Design review of the part built by this model. Coordinates are the model's own, in mm. A direction names the side the tool comes from. Give positions to 0.01 mm unless a question says otherwise; leave off trailing zeros. Order: outer loops, then holes, each group sorted by start corner. A loop starts at its lowest first (then second) coordinate and runs counter-clockwise, first axis right, second up. Notation, with made-up numbers: M 16.25,60.25 L 50.25,60.25 A18 ccw 50.25,69.25 Z; hole C 14.5,85.5 d8. An arc over 180 degrees is marked long. Answer as a JSON object with one key per item and string values.
from build123d import *

# Parameters (mm, degrees)
SKETCH1_R           = 30
SKETCH1_R_2         = 7
BOSS_EXTRUDE1_DEPTH = 10
CUT_EXTRUDE1_DEPTH  = 21
FILLET1_R           = 30
FILLET2_R           = 55


with BuildPart() as part:
    # Sketch1 → Boss-Extrude1 (new body, symmetric)
    with BuildSketch(Plane(origin=(0, 0, 0), x_dir=(1, 0, 0), z_dir=(0, 1, 0))):
        with BuildLine():
            Line((128.063755469, 9.084385863), (27.935473676, 25.760615491))
            ThreePointArc((27.935473676, 25.760615491), (-38, 0), (27.935473676, -25.760615491))
            Line((27.935473676, -25.760615491), (128.063755469, -9.084385863))
            ThreePointArc((128.063755469, -9.084385863), (155, 0), (128.063755469, 9.084385863))
        make_face()
        Circle(SKETCH1_R, mode=Mode.SUBTRACT)
        with Locations((140, 0)):
            Circle(SKETCH1_R_2, mode=Mode.SUBTRACT)
    extrude(amount=BOSS_EXTRUDE1_DEPTH, both=True)

    # Sketch2 → Cut-Extrude1 (cut, through all)
    with BuildSketch(Plane(origin=(0, 10, 0), x_dir=(1, 0, 0), z_dir=(0, 1, 0))):
        with BuildLine():
            Line((44.461373165, 15.911828816), (101.502639752, 6.411683174))
            ThreePointArc((101.502639752, 6.411683174), (106.934782609, 0), (101.502639752, -6.411683174))
            Line((101.502639752, -6.411683174), (44.461373165, -15.911828816))
            ThreePointArc((44.461373165, -15.911828816), (39.963398771, -14.368423983), (38.791061861, -9.759790965))
            ThreePointArc((38.791061861, -9.759790965), (40, 0), (38.791061861, 9.759790965))
            ThreePointArc((38.791061861, 9.759790965), (39.963398771, 14.368423983), (44.461373165, 15.911828816))
        make_face()
    extrude(amount=-CUT_EXTRUDE1_DEPTH, mode=Mode.SUBTRACT)

    # Fillet1
    fillet1_edges = [part.edges().sort_by_distance(p)[0] for p in [
        (128.063755469, 0, 9.084385863),
        (128.063755469, 0, -9.084385863),
    ]]
    fillet(fillet1_edges, radius=FILLET1_R)

    # Fillet2
    fillet2_edges = [part.edges().sort_by_distance(p)[0] for p in [
        (27.935473676, 0, 25.760615491),
        (27.935473676, 0, -25.760615491),
    ]]
    fillet(fillet2_edges, radius=FILLET2_R)


solid = part.part
(1) Insertion check: pin 1 (4 mm diameter, centred on x = 29, y = 5, fed in from -Z); pin 2 (5 mm diameter, centred on x = 71, y = 6.5, fed in from -Z); pin 3 (1 mm diameter, centred on y = 2, z = 21, fed in from -X). Each pin has a flat end and moves straight along its axis. Give the tip position at first contact, or say it passes through.
Checked values:
{"pin 1": "stops at z = -28.25", "pin 2": "stops at z = -19", "pin 3": "stops at x = -32"}
(2) We need section C-C (y = -8). Write out the cut boundary in (x, z).
Checked values:
{"outline": "M 20.92,-31.73 A55 cw 42.15,-23.39 L 115.89,-11.11 A30 cw 133.6,-13.57 A15 ccw long 133.6,13.57 A30 cw 115.89,11.11 L 42.15,23.39 A55 cw 20.92,31.73 A38 ccw long Z; hole C 0,0 d60; hole M 38.79,-9.76 A5 ccw 44.46,-15.91 L 101.5,-6.41 A6.5 ccw 101.5,6.41 L 44.46,15.91 A5 ccw 38.79,9.76 A40 cw Z; hole C 140,0 d14"}
(3) Draft analysis for pull direction X (two halves, no side actions). For faces 4 (the cylindrical face through (-37.983, 0.14, -1.146)), 5 (the flat face through (58, 10, -14)), 6 (the flat face through (78.5, 0.14, 17.34)), state which applies: +X half, -X half, draft (parallel to the pull), parting line (faces both ways), or undercut.
Checked values:
{"face 4": "parting line", "face 5": "draft", "face 6": "undercut"}
(4) We need section D-D (z = 18.5). Write out the cut boundary in (x, y).
Checked values:
{"outline": "M -33.19,-10 L -23.62,-10 L -23.62,10 L -33.19,10 Z; M 23.62,-10 L 71.53,-10 L 71.53,10 L 23.62,10 Z"}
(5) Tool access review of faces 1 (the cylindrical face through (106.934, 0.14, -0.128)), 2 (the cylindrical face through (125, 0, 11)), 3 (the flat face through (79.535, 0.14, -17.167)): name each direction out of +Z, -Z, +X, -X, +Y, -Y from which nothing blocks a thin tool from reaching the whole face with its end or side.
Checked values:
{"face 1": "+Y, -Y", "face 2": "+Z, +Y, -Y", "face 3": "-Z, +Y, -Y"}
(6) We need section A-A (x = 0). Write out the cut boundary in (y, z).
Checked values:
{"outline": "M -10,-38 L 10,-38 L 10,-30 L -10,-30 Z; M -10,30 L 10,30 L 10,38 L -10,38 Z"}
(7) We need section B-B (z = 0). Write out the cut boundary in (x, y).
Checked values:
{"outline": "M -38,-10 L -30,-10 L -30,10 L -38,10 Z; M 30,-10 L 40,-10 L 40,10 L 30,10 Z; M 106.93,-10 L 133,-10 L 133,10 L 106.93,10 Z; M 147,-10 L 155,-10 L 155,10 L 147,10 Z"}
(8) To check wall thickness, follow L1, parallel to X at y = -5.5, z = 0; L2, parallel to Z at x = 140, y = 2.75; L3, parallel to Z at x = 0, y = -2.75. State the ranges of each line that lie inside material, in increasing order. Write a range as from..to.
Checked values:
{"L1": "x = -38..-30, 30..40, 106.93..133, 147..155", "L2": "z = -15..-7, 7..15", "L3": "z = -38..-30, 30..38"}
